from build123d import *

# Parameters (mm, degrees)
SKETCH1_W           = 15
SKETCH1_H           = 6
SKETCH1_W_2         = 8
SKETCH1_H_2         = 20
BOSS_EXTRUDE1_DEPTH = 14
SKETCH3_W           = 15
SKETCH3_H           = 6
SKETCH3_W_2         = 8
SKETCH3_H_2         = 20
BOSS_EXTRUDE2_DEPTH = 6.5
FILLET1_R           = 4
SKETCH4_R           = 2
SKETCH4_R_2         = 5.5
BOSS_EXTRUDE3_DEPTH = 6
SKETCH5_R           = 12.05
CUT_EXTRUDE1_DEPTH  = 3


with BuildPart() as part:
    # Sketch1 → Boss-Extrude1 (new body)
    # profile 1 of 6: a face of its own
    with BuildSketch(Plane.XY):
        Polygon((-4, -9), (4, -9), (45, -9), (45, 9), (-45, 9), (-45, -9), align=None)
        with Locations((-15, 0)):
            Rectangle(SKETCH1_W, SKETCH1_H, mode=Mode.SUBTRACT)
        with Locations((15, 0)):
            Rectangle(SKETCH1_W, SKETCH1_H, mode=Mode.SUBTRACT)
    # profile 2 of 6: a face of its own
    with BuildSketch(Plane.XY):
        with Locations((0, -19)):
            Rectangle(SKETCH1_W_2, SKETCH1_H_2)
    # profile 3 of 6: a face of its own
    with BuildSketch(Plane.XY):
        with Locations((-15, 0)):
            Rectangle(SKETCH1_W, SKETCH1_H)
    # profile 4 of 6: a face of its own
    with BuildSketch(Plane.XY):
        with Locations((15, 0)):
            Rectangle(SKETCH1_W, SKETCH1_H)
    # profile 5 of 6: a face of its own
    with BuildSketch(Plane.XY):
        Polygon((45, -9), (4, -9), (4, -19), align=None)
    # profile 6 of 6: a face of its own
    with BuildSketch(Plane.XY):
        Polygon((-4, -19), (-4, -9), (-45, -9), align=None)
    extrude(amount=BOSS_EXTRUDE1_DEPTH)

    # Sketch3 → Boss-Extrude2 (add)
    # profile 1 of 2: a face of its own
    with BuildSketch(Plane.XY):
        Polygon((-4, -9), (4, -9), (45, -9), (45, 9), (-45, 9), (-45, -9), align=None)
        with Locations((-15, 0)):
            Rectangle(SKETCH3_W, SKETCH3_H, mode=Mode.SUBTRACT)
        with Locations((15, 0)):
            Rectangle(SKETCH3_W, SKETCH3_H, mode=Mode.SUBTRACT)
    # profile 2 of 2: a face of its own
    with BuildSketch(Plane.XY):
        with Locations((0, -19)):
            Rectangle(SKETCH3_W_2, SKETCH3_H_2)
    extrude(amount=-BOSS_EXTRUDE2_DEPTH)

    # Fillet1
    fillet1_edges = [part.edges().sort_by_distance(p)[0] for p in [
        (-4, -29, 3.75),
        (4, -29, 3.75),
    ]]
    fillet(fillet1_edges, radius=FILLET1_R - 0.0001)  # a hair under: the kernel refuses the full size

    # Sketch4 → Boss-Extrude3 (add)
    with BuildSketch(Plane.XY.offset(14)):
        with BuildLine():
            Line((13.964514824, 9), (13.964514824, 46.5))
            ThreePointArc((13.964514824, 46.5), (0, 60.464514824), (-13.964514824, 46.5))
            Line((-13.964514824, 46.5), (-13.964514824, 9))
            Line((-13.964514824, 9), (13.964514824, 9))
        make_face()
        with Locations((8.5, 46.5)):
            Circle(SKETCH4_R, mode=Mode.SUBTRACT)
        with Locations((-8.5, 46.5)):
            Circle(SKETCH4_R, mode=Mode.SUBTRACT)
        with Locations((0, 46.5)):
            Circle(SKETCH4_R_2, mode=Mode.SUBTRACT)
    extrude(amount=-BOSS_EXTRUDE3_DEPTH)

    # Sketch5 → Cut-Extrude1 (cut)
    with BuildSketch(Plane(origin=(0, 0, 8), x_dir=(-1, 0, 0), z_dir=(0, 0, -1))):
        with Locations((0, 46.5)):
            Circle(SKETCH5_R)
    extrude(amount=-CUT_EXTRUDE1_DEPTH, mode=Mode.SUBTRACT)


solid = part.part
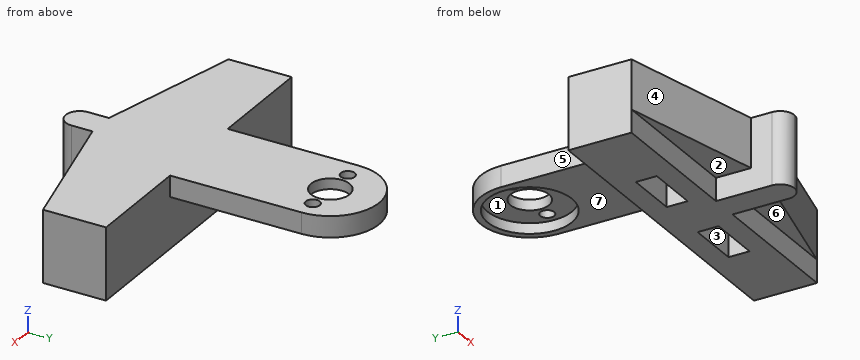
Read the model definition and answer for the solid it produces. Units are mm, in the model's axes. Face numbers are marked on the shaded views. A direction names the side the tool comes from. Give positions to 0.01 mm unless a question says otherwise; leave off trailing zeros. Write each loop counter-clockwise with the first axis right and the second up, starting at its lowest first coordinate (ties: lowest second). Pieces come first, ordered by that corner, then holes. Notation, with made-up numbers: (20.25, -17) - (76.25, -17) arc R17 cw to (76.25, -5) - close; hole circle Ø8 at (18, -29.75). An arc over 180 degrees is marked (long way). Answer in a Markdown table with one row per item. Add a question column.
Item 1: Section B-B, the plane y = -11.5 is taken. Write down the section's boundary in (x, z).
Item 2: Determine the mould class of the marked faces 1, 2, 3 and 4 for opening direction X: pulls with the +X half, pulls with the -X half, needs draft (parallel to the pull), parting line crosses it, or undercut.
Item 3: Section D-D, the plane x = 37 is taken. Write down the section's boundary in (y, z), and give its area (3 significant figures).
Item 4: Section A-A, the plane z = -1.75 is taken. Count the separate pieces of the cut face and the enclosed holes in it, and give its area (3 significant figures).
Item 5: A tool of negligible diameter and unlimited length cuts with its end or side. For the marked faces 5, 6 and 7, from which of +Z, -Z, +X, -X, +Y, -Y can it reach the whole face along a straight path? Write none if from no direction.
Item 6: Find the intervals of material crossed by L1, parallel to Y at x = 0, z = 8.9; L2, parallel to Y at x = 18, z = -1.5; L3, parallel to X at y = 39.5, z = 12, in increasing order.
Item 7: Flat-ended cylindrical pins translate along their axes: P1, Ø7, axis at x = -16.5, z = -3.5, coming from the +Y side; P2, Ø5, axis at y = 27, z = 10, coming from the -X side; P3, Ø3, axis at x = -32, z = 3.5, coming from the -Y side. Find the tip coordinate at first contact, or state that the pin passes through.
Recorded:
| question | item | result |
|---|---|---|
| 1 | outline | (-34.75, 0) - (-4, 0) - (-4, -6.5) - (4, -6.5) - (4, 0) - (34.75, 0) - (34.75, 14) - (-34.75, 14) - close |
| 2 | face 1 | undercut |
| 2 | face 2 | needs draft |
| 2 | face 3 | undercut |
| 2 | face 4 | pulls with the -X half |
| 3 | outline | (-10.95, 0) - (-9, 0) - (-9, -6.5) - (9, -6.5) - (9, 14) - (-10.95, 14) - close |
| 3 | area | 396 mm2 |
| 4 | separate pieces | 1 |
| 4 | enclosed holes | 2 |
| 4 | area | 1,590 mm2 |
| 5 | face 5 | +Z, -Z, -X, +Y |
| 5 | face 6 | -Z, +X, -Y |
| 5 | face 7 | -Z, +X, -X, +Y |
| 6 | L1 | y = -29 to 34.45, 58.55 to 60.46 |
| 6 | L2 | y = -9 to -3, 3 to 9 |
| 6 | L3 | x = -13.96 to 13.96 |
| 7 | P1 | stops at y = 9 |
| 7 | P2 | stops at x = -13.96 |
| 7 | P3 | stops at y = -12.54 |
